from build123d import *

# Parameters (mm, degrees)
SKETCH005_W     = 19
SKETCH005_H     = 2
PAD004_DEPTH    = 10
FILLET003_R     = 1
CHAMFER005_SIZE = 0.5


with BuildPart() as part:
    # Sketch005 → Pad004 (new body)
    with BuildSketch(Plane.YZ):
        with Locations((-9.5, 1)):
            Rectangle(SKETCH005_W, SKETCH005_H)
    extrude(amount=PAD004_DEPTH)

    # Fillet003
    fillet003_edges = [part.edges().sort_by_distance(p)[0] for p in [
        (5, -19, 2),
        (0, -19, 1),
        (0, -9.5, 2),
        (10, -9.5, 2),
        (0, 0, 1),
        (10, -19, 1),
    ]]
    fillet(fillet003_edges, radius=FILLET003_R)

    # Chamfer005
    chamfer005_edges = [part.edges().sort_by_distance(p)[0] for p in [
        (10, -9, 0),
    ]]
    chamfer(chamfer005_edges, length=CHAMFER005_SIZE)


with BuildPart() as part_1:
    # Body005 placement: moved
    add(part.part.moved(Location((3.8, 17.5, -4.7))))


solid = part_1.part
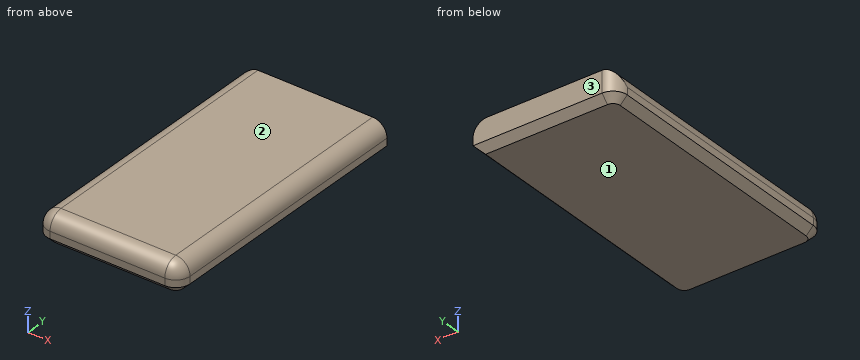
Check sheet for the modelled part. Datum: model origin and axes. Units: mm. Face numbers are marked on the shaded views. Round coordinates to 2 decimals unless told otherwise and drop trailing zeros. Order: outer loops, then holes, each group sorted by start corner. A loop starts at its lowest first (then second) coordinate and runs counter-clockwise, first axis right, second up. Notation, with made-up numbers: M -5.75,14 L 50.25,14 A16 cw 50.25,44 Z; hole C -10,31.25 d5. An arc over 180 degrees is marked long. One line per item, written item: value. Start each with the question number.
1. Section check B-B on z = -3.05. Enter the section's corners in (x, y), and give its area (3 significant figures).
2. Release check for a two-part mould opening along Z. For the marked faces 1, 2 and 3 record: released by +Z, released by -Z, zero draft, split by the parting line, or undercut.
3. Gauge pin test, flat end, axial feed: P1, Ø1, axis at y = 0.5, z = -3.5, coming from the -X side. Record the tip position at first contact, or that the pin passes through.
4. Section check A-A on y = 10.5. Enter the section's corners in (x, z).
5. Scan lines: line 1 along Y through (x, z) = (9.5, -3.65); line 2 along Z through (x, y) = (4.5, 0.75); line 3 along Y through (x, z) = (12, -3.15). Record each from-to range of solid material in increasing order.
Results found:
1. outline: M 4.04,-0.5 A0.76 ccw 4.8,-1.26 L 12.8,-1.26 A0.76 ccw 13.56,-0.5 L 13.56,17.5 L 4.8,17.5 A1 ccw 4.04,17.15 Z
1. area: 178 mm^2
2. face 1: released by -Z
2. face 2: released by +Z
2. face 3: zero draft
3. P1: x = 3.8
4. outline: M 3.8,-4.2 L 4.3,-4.7 L 13.3,-4.7 L 13.8,-4.2 L 13.8,-3.7 A1 ccw 12.8,-2.7 L 4.8,-2.7 A1 ccw 3.8,-3.7 Z
5. line 1: -1.5 to 17.5
5. line 2: -4.7 to -2.75
5. line 3: -1.34 to 17.5
